Read the model definition and answer for the solid it produces. Units are mm, in the model's axes. Face numbers are marked on the shaded views. A direction names the side the tool comes from. Round coordinates to 2 decimals unless told otherwise and drop trailing zeros. Write each loop counter-clockwise with the first axis right and the second up, starting at its lowest first coordinate (ties: lowest second). Pieces come first, ordered by that corner, then holes. Notation, with made-up numbers: (74.5, 74.5) - (133.5, 74.5) arc R8 cw to (133.5, 80.5) - close; hole circle Ø4 at (-8.5, -10). An arc over 180 degrees is marked (long way). Answer as CSV lines item,"result". Start each with the question number.
1) Find section D-D on x = -6.5. Determine the outline of the cut face in (y, z).
2) Find section A-A on z = -11.75. Determine the outline of the cut face in (x, y).
3) Find section C-C on y = 4.25. Determine the outline of the cut face in (x, z).
4) Consider line 1 along Z through (x, y) = (18.5, 2.5); line 2 along Z through (x, y) = (11, -3); line 3 along X through (y, z) = (3, -10.25). Determine where each line is inside the solid, lowest interval first.
5) Each of these flat-tipped pins is pushed along its axis until it touches: pin 1 (3.5 mm diameter, centred on y = 3, z = -17, fed in from +X); pin 2 (2.5 mm diameter, centred on x = 13, y = -2, fed in from +Z); pin 3 (1 mm diameter, centred on x = 11, y = -1, fed in from -Z); pin 4 (4 mm diameter, centred on x = -5, z = -9, fed in from -Y). Where does it stop, or does it pass through?
6) Find section B-B on x = 17.5. Determine the outline of the cut face in (y, z), then the cut area to 3 significant figures.
7) Which of the six approach directions +Z, -Z, +X, -X, +Y, -Y give full straight-line access (tool end or side, diameter ignored) to the marked faces 1, 2, 3 and 4?
from build123d import *

# Parameters (mm, degrees)
SKETCH1_W           = 27.2034
SKETCH1_H           = 27.2034
BOSS_EXTRUDE1_DEPTH = 0.8128
BOSS_EXTRUDE2_DEPTH = 4.2164
BOSS_EXTRUDE3_DEPTH = 3.2512
SKETCH4_R           = 1.4351
BOSS_EXTRUDE4_DEPTH = 12.7


with BuildPart() as part:
    # Sketch1 → Boss-Extrude1 (new body)
    with BuildSketch(Plane(origin=(0, 0, 0), x_dir=(1, 0, 0), z_dir=(0, 1, 0))):
        with Locations((13.6017, 13.6017)):
            Rectangle(SKETCH1_W, SKETCH1_H)
    extrude(amount=BOSS_EXTRUDE1_DEPTH)

    # Sketch2 → Boss-Extrude2 (add)
    with BuildSketch(Plane(origin=(0, 0.8128, 0), x_dir=(1, 0, 0), z_dir=(0, 1, 0))):
        with BuildLine():
            Line((3.1303, 26.0731), (24.0731, 26.0731))
            ThreePointArc((24.0731, 26.0731), (25.487313562, 25.487313562), (26.0731, 24.0731))
            Line((26.0731, 24.0731), (26.0731, 3.1303))
            ThreePointArc((26.0731, 3.1303), (25.487313562, 1.716086438), (24.0731, 1.1303))
            Line((24.0731, 1.1303), (3.1303, 1.1303))
            ThreePointArc((3.1303, 1.1303), (1.716086438, 1.716086438), (1.1303, 3.1303))
            Line((1.1303, 3.1303), (1.1303, 24.0731))
            ThreePointArc((1.1303, 24.0731), (1.716086438, 25.487313562), (3.1303, 26.0731))
        make_face()
    extrude(amount=BOSS_EXTRUDE2_DEPTH)

    # Sketch3 → Boss-Extrude3 (add)
    with BuildSketch(Plane.XZ):
        Polygon((23.771814156, -1.5367), (3.431585844, -1.5367), (1.5367, -3.431585844), (1.5367, -23.771814156), (3.431585844, -25.6667), (23.771814156, -25.6667), (25.6667, -23.771814156), (25.6667, -3.431585844), align=None)
    extrude(amount=BOSS_EXTRUDE3_DEPTH)

    # Sketch4 → Boss-Extrude4 (add)
    with BuildSketch(Plane.ZY.offset(-1.5367)):
        with Locations((-13.6017, -1.6256)):
            Circle(SKETCH4_R)
    extrude(amount=BOSS_EXTRUDE4_DEPTH)


solid = part.part
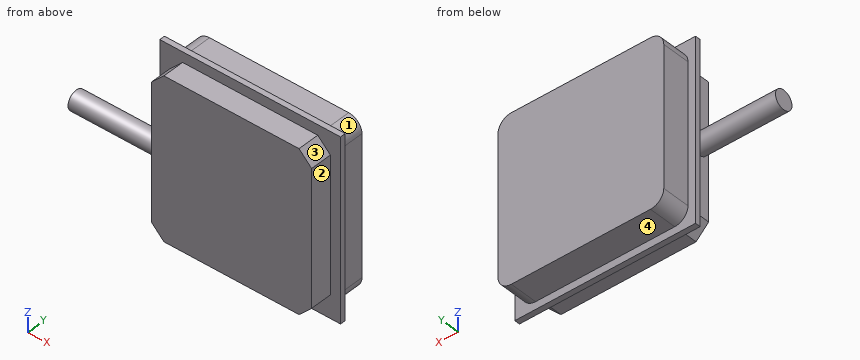
Check values:
1,outline,"circle Ø2.87 at (-1.63, -13.6)"
2,outline,"(0, 0) - (1.54, 0) - (1.54, -3.25) - (25.67, -3.25) - (25.67, 0) - (27.2, 0) - (27.2, 0.81) - (26.07, 0.81) - (26.07, 5.03) - (1.13, 5.03) - (1.13, 0.81) - (0, 0.81) - close"
3,outline,"(1.13, -24.07) arc R2 ccw to (3.13, -26.07) - (24.07, -26.07) arc R2 ccw to (26.07, -24.07) - (26.07, -3.13) arc R2 ccw to (24.07, -1.13) - (3.13, -1.13) arc R2 ccw to (1.13, -3.13) - close"
4,line 1,"z = -26.07 to -1.13"
4,line 2,"z = -25.67 to -1.54"
4,line 3,"x = 1.13 to 26.07"
5,pin 1,"stops at x = 26.07"
5,pin 2,"stops at z = -1.54"
5,pin 3,"stops at z = -25.67"
5,pin 4,"passes through"
6,outline,"(-3.25, -25.67) - (0, -25.67) - (0, -27.2) - (0.81, -27.2) - (0.81, -26.07) - (5.03, -26.07) - (5.03, -1.13) - (0.81, -1.13) - (0.81, 0) - (0, 0) - (0, -1.54) - (-3.25, -1.54) - close"
6,area,"206 mm^2"
7,face 1,"+Z, +X, +Y"
7,face 2,"+Z, -Z, +X, -Y"
7,face 3,"+Z, +X, -Y"
7,face 4,"-Z, +X, -X, +Y"
